Work out the finished part from the listing and answer in its coordinate system (mm). Face numbers are marked on the shaded views. A direction names the side the tool comes from. Round coordinates to 2 decimals unless told otherwise and drop trailing zeros. Order: outer loops, then holes, each group sorted by start corner. A loop starts at its lowest first (then second) coordinate and runs counter-clockwise, first axis right, second up. Notation, with made-up numbers: (79, 16) -> (102, 16) arc R32 cw to (102, 53) -> close; hole circle Ø11 at (-13, -34.5). An arc over 180 degrees is marked (long way). Use a Markdown table: item, result. Add a question column.
Item 1: Flat-ended cylindrical pins translate along their axes: P1, Ø4, axis at x = 18.5, z = -15, coming from the +Y side; P2, Ø5.5, axis at x = 22, z = -2, coming from the -Y side; P3, Ø3, axis at x = 5, y = 5.5, coming from the +Z side. Find the tip coordinate at first contact, or state that the pin passes through.
Item 2: For a pull along Z with two mould halves and no side action, classify the marked faces 6, 7, 8 and 9 as +Z half, -Z half, draft (parallel to the pull), parting line (faces both ways), or undercut.
Item 3: A cutting plane is placed at A-A, the plane z = -15.25. Determine the outline of the cut face in (x, y).
Item 4: A cutting plane is placed at B-B, the plane x = 20. Determine the outline of the cut face in (y, z).
Item 5: A cutting plane is placed at C-C, the plane y = 0. Give the number of separate pieces and of enclosed holes in the cut face, plus the area to 3 significant figures.
Item 6: A tool of negligible diameter and unlimited length cuts with its end or side. For the marked faces 1, 2, 3, 4 and 5, from which of +Z, -Z, +X, -X, +Y, -Y can it reach the whole face along a straight path? Write none if from no direction.
Item 7: Find the intervals of material crossed by L1, parallel to X at y = -1.5, z = -15; L2, parallel to Y at x = 17, z = 0; L3, parallel to X at y = 2.25, z = 13.5, in increasing order. Write a range as [from, to].
from build123d import *

# Parameters (mm, degrees)
SKETCH1_R           = 11
BOSS_EXTRUDE1_DEPTH = 36
EXTRUDE_THIN1_START = 0.5
SKETCH1_4_R         = 6.5
SKETCH1_4_R_2       = 6
EXTRUDE_THIN1_DEPTH = 29.5
BOSS_EXTRUDE2_START = 0.8
SKETCH1_5_R         = 10
SKETCH1_5_R_2       = 6
BOSS_EXTRUDE2_DEPTH = 29
BOSS_EXTRUDE3_START = 0.3
SKETCH1_6_R         = 11
SKETCH1_6_R_2       = 10
BOSS_EXTRUDE3_DEPTH = 31
BOSS_EXTRUDE4_START = 1
BOSS_EXTRUDE4_DEPTH = 1
FILLET1_R           = 0.5
SKETCH4_R           = 2.15
CUT_EXTRUDE3_DEPTH  = 51.209560914
CHAMFER1_SIZE       = 1


with BuildPart() as part:
    # Sketch1 → Boss-Extrude1 (new body)
    with BuildSketch(Plane(origin=(0, 0, 0), x_dir=(0, 0, -1), z_dir=(1, 0, 0))):
        Polygon((-21, -7), (-19.5, -5.5), (-19.5, 9), (-11, 9), (-5, 13), (5, 13), (11, 9), (19.5, 9), (19.5, -5.5), (21, -7), (21, -15), (11, -15), (9.5, -13.5), (-9.5, -13.5), (-11, -15), (-21, -15), align=None)
        Circle(SKETCH1_R, mode=Mode.SUBTRACT)
    extrude(amount=BOSS_EXTRUDE1_DEPTH)



with BuildPart() as body_2:
    # Sketch1_4 → Extrude-Thin1 (new body)
    with BuildSketch(Plane(origin=(0, 0, 0), x_dir=(0, 0, -1), z_dir=(1, 0, 0)).offset(EXTRUDE_THIN1_START)):
        Circle(SKETCH1_4_R)
        Circle(SKETCH1_4_R_2, mode=Mode.SUBTRACT)
    extrude(amount=EXTRUDE_THIN1_DEPTH)

    # Sketch1_5 → Boss-Extrude2 (add)
    with BuildSketch(Plane(origin=(0, 0, 0), x_dir=(0, 0, -1), z_dir=(1, 0, 0)).offset(BOSS_EXTRUDE2_START)):
        with Locations(Location((0, 0, 0), (0, 0, 180))):
            Circle(SKETCH1_5_R)
        Circle(SKETCH1_5_R_2, mode=Mode.SUBTRACT)
    extrude(amount=BOSS_EXTRUDE2_DEPTH)


with BuildPart() as part_1:
    add(part.part)

    add(body_2.part)  # Boss-Extrude3 merges body 2
    # Sketch1_6 → Boss-Extrude3 (add)
    with BuildSketch(Plane(origin=(0, 0, 0), x_dir=(0, 0, -1), z_dir=(1, 0, 0)).offset(BOSS_EXTRUDE3_START)):
        Circle(SKETCH1_6_R)
        Circle(SKETCH1_6_R_2, mode=Mode.SUBTRACT)
    extrude(amount=BOSS_EXTRUDE3_DEPTH)

    # Sketch3 → Boss-Extrude4 (add)
    with BuildSketch(Plane(origin=(31.3, 0, 0), x_dir=(0, 0, -1), z_dir=(1, 0, 0)).offset(BOSS_EXTRUDE4_START)):
        with BuildLine():
            Line((-1.011429614, -9.94871902), (-1.112572576, -10.943590922))
            ThreePointArc((-1.112572576, -10.943590922), (0, 11), (1.112572576, -10.943590922))
            Line((1.112572576, -10.943590922), (1.011429614, -9.94871902))
            ThreePointArc((1.011429614, -9.94871902), (1.535872296, -8.912190675), (2.686623353, -9.070945649))
            ThreePointArc((2.686623353, -9.070945649), (4.301522401, -8.715825098), (3.378506843, -7.343946161))
            ThreePointArc((3.378506843, -7.343946161), (0, 8.083801933), (-3.378506843, -7.343946161))
            ThreePointArc((-3.378506843, -7.343946161), (-4.301522401, -8.715825098), (-2.686623353, -9.070945649))
            ThreePointArc((-2.686623353, -9.070945649), (-1.535872296, -8.912190675), (-1.011429614, -9.94871902))
        make_face()
    extrude(amount=BOSS_EXTRUDE4_DEPTH)

    # Fillet1
    fillet1_edges = [part_1.edges().sort_by_distance(p)[0] for p in [
        (36, -6.25, 20.25),
        (36, -11, 21),
        (0, 1.75, 19.5),
        (0, 9, 15.25),
        (0, 11, 8),
        (0, 13, 0),
        (0, 11, -8),
        (0, 9, -15.25),
        (0, 1.75, -19.5),
        (0, -6.25, -20.25),
        (0, -11, -21),
        (0, -11, 21),
        (0, -6.25, 20.25),
        (18, -5.5, 19.5),
        (18, 9, 19.5),
        (18, 9, 11),
        (18, 13, 5),
        (18, 13, -5),
        (18, 9, -11),
        (18, 9, -19.5),
        (18, -5.5, -19.5),
        (18, -7, -21),
        (18, -7, 21),
        (36, -11, -21),
        (36, -6.25, -20.25),
        (36, 1.75, -19.5),
        (36, 9, -15.25),
        (36, 11, -8),
        (36, 13, 0),
        (36, 11, 8),
        (36, 9, 15.25),
        (36, 1.75, 19.5),
    ]]
    fillet(fillet1_edges, radius=FILLET1_R)

    # Sketch4 → Cut-Extrude3 (cut, through all)
    with BuildSketch(Plane.XZ.offset(15)):
        with Locations(Location((5, 15.25, 0), (0, 0, 270))):
            Circle(SKETCH4_R)
        with Locations(Location((31, 15.25, 0), (0, 0, 270))):
            Circle(SKETCH4_R)
        with Locations(Location((31, -15.25, 0), (0, 0, 270))):
            Circle(SKETCH4_R)
        with Locations(Location((5, -15.25, 0), (0, 0, 270))):
            Circle(SKETCH4_R)
    extrude(amount=-CUT_EXTRUDE3_DEPTH, mode=Mode.SUBTRACT)

    # Chamfer1
    chamfer1_edges = [part_1.edges().sort_by_distance(p)[0] for p in [
        (5, 9, -13.1),
        (31, 9, -13.1),
        (31, 9, 17.4),
        (31, -15, 17.4),
        (5, 9, 17.4),
        (5, -15, 17.4),
    ]]
    chamfer(chamfer1_edges, length=CHAMFER1_SIZE)


solid = part_1.part
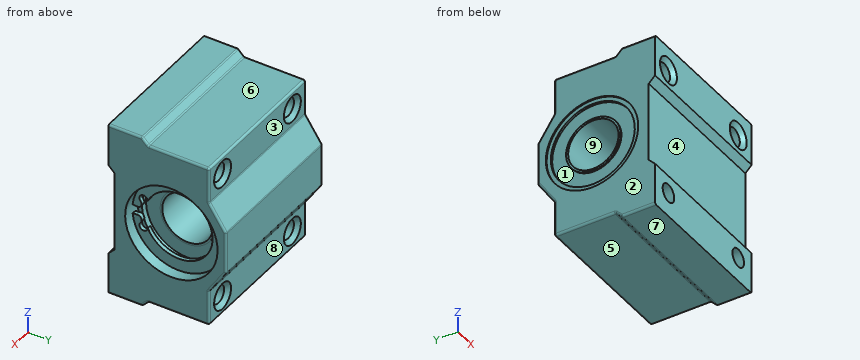
Reported:
| question | item | result |
|---|---|---|
| 1 | P1 | y = 9 |
| 1 | P2 | y = -13.5 |
| 1 | P3 | z = 19.5 |
| 2 | face 6 | +Z half |
| 2 | face 7 | -Z half |
| 2 | face 8 | draft |
| 2 | face 9 | undercut |
| 3 | outline | (0, -15) -> (2.85, -15) -> (2.85, 8) -> (1.85, 9) -> (0.5, 9) arc R0.5 ccw to (0, 8.5) -> close; (7.15, -15) -> (28.85, -15) -> (28.85, 8) -> (27.85, 9) -> (8.15, 9) -> (7.15, 8) -> close; (33.15, -15) -> (36, -15) -> (36, 8.5) arc R0.5 ccw to (35.5, 9) -> (34.15, 9) -> (33.15, 8) -> close |
| 4 | outline | (-15, -21) -> (-7.21, -21) arc R0.5 ccw to (-6.85, -20.85) -> (-5.65, -19.65) arc R0.5 cw to (-5.29, -19.5) -> (8.5, -19.5) arc R0.5 ccw to (9, -19) -> (9, -11.15) arc R0.5 cw to (9.08, -10.87) -> (12.92, -5.13) arc R0.5 ccw to (13, -4.85) -> (13, 4.85) arc R0.5 ccw to (12.92, 5.13) -> (9.08, 10.87) arc R0.5 cw to (9, 11.15) -> (9, 19) arc R0.5 ccw to (8.5, 19.5) -> (-5.29, 19.5) arc R0.5 cw to (-5.65, 19.65) -> (-6.85, 20.85) arc R0.5 ccw to (-7.21, 21) -> (-15, 21) -> (-15, 11) -> (-13.5, 9.5) -> (-13.5, -9.5) -> (-15, -11) -> close; hole circle Ø12 at (0, 0) |
| 5 | separate pieces | 2 |
| 5 | enclosed holes | 4 |
| 5 | area | 854 mm² |
| 6 | face 1 | -X |
| 6 | face 2 | +Z, -Z, -X, +Y, -Y |
| 6 | face 3 | +Z, +X, -X, +Y |
| 6 | face 4 | +X, -X, -Y |
| 6 | face 5 | -Z, +X, -X, +Y |
| 7 | L1 | [0, 2.86], [7.14, 28.86], [33.14, 36] |
| 7 | L2 | [-13.5, -6], [6, 13] |
| 7 | L3 | [0, 3.75], [6.25, 29.75], [32.25, 36] |
